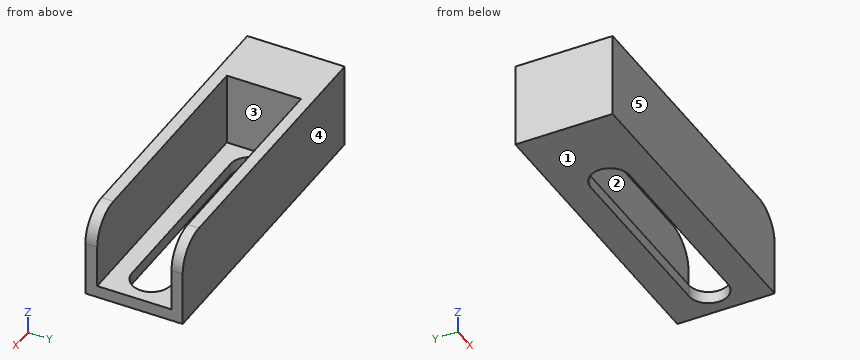
from build123d import *

# Parameters (mm, degrees)
SKETCH_W        = 50
SKETCH_H        = 16
PAD_DEPTH       = 14
SKETCH001_W     = 40
SKETCH001_H     = 12.2
POCKET_DEPTH    = 12
POCKET001_DEPTH = 5
FILLET_R        = 5


with BuildPart() as part:
    # Sketch → Pad (new body)
    with BuildSketch(Plane.XY):
        with Locations((25, 8)):
            Rectangle(SKETCH_W, SKETCH_H)
    extrude(amount=PAD_DEPTH)

    # Sketch001 (on Face6 of Pad) → Pocket (cut)
    with BuildSketch(Plane.XY.offset(14)):
        with Locations((30, 8.058537)):
            Rectangle(SKETCH001_W, SKETCH001_H)
    extrude(amount=-POCKET_DEPTH, mode=Mode.SUBTRACT)

    # Sketch002 (on Face8 of Pocket) → Pocket001 (cut)
    with BuildSketch(Plane.XY.offset(2)):
        with BuildLine():
            ThreePointArc((14.443499, 11.3), (11.243499, 8.1), (14.443499, 4.9))
            Line((14.443499, 4.9), (44.78962, 4.9))
            ThreePointArc((44.78962, 4.9), (47.98962, 8.1), (44.78962, 11.3))
            Line((14.443499, 11.3), (44.78962, 11.3))
        make_face()
    extrude(amount=-POCKET001_DEPTH, mode=Mode.SUBTRACT)

    # Fillet
    fillet_edges = [part.edges().sort_by_distance(p)[0] for p in [
        (50, 0.979269, 14),
        (50, 15.079269, 14),
    ]]
    fillet(fillet_edges, radius=FILLET_R)


solid = part.part
Part model, mm, in its own coordinate system. Face numbers are marked on the shaded views. A direction names the side the tool comes from. Give positions to 0.01 mm unless a question says otherwise; leave off trailing zeros. Order: outer loops, then holes, each group sorted by start corner. A loop starts at its lowest first (then second) coordinate and runs counter-clockwise, first axis right, second up. Notation, with made-up numbers: (-6, -16.75) - (52, -16.75) arc R20 ccw to (52, 16.25) - close; hole circle Ø3 at (19, 81). An arc over 180 degrees is marked (long way). Use a Markdown table: item, result.
1) Two-plate mould, pull along Y, no slides. Class the marked faces 3, 4 and 5: +Y half, -Y half, draft (parallel to the pull), parting line (faces both ways), or undercut.
Checked values:
| item | result |
|---|---|
| face 3 | undercut |
| face 4 | +Y half |
| face 5 | -Y half |
2) Probe L1, parallel to Y at x = 14, z = 9; L2, parallel to X at y = 5, z = 8; L3, parallel to Z at x = 30, y = 2. List the from-to ranges inside material, lowest first. Write a range as from..to.
Checked values:
| item | result |
|---|---|
| L1 | 0..1.96, 14.16..16 |
| L2 | 0..10 |
| L3 | 0..2 |
3) 3-axis set-ups, long thin cutter, end or side, ignore diameter. For the marked faces 1 and 2: which of +Z, -Z, +X, -X, +Y, -Y reach the whole face in a straight line?
Checked values:
| item | result |
|---|---|
| face 1 | -Z, +X, -X, +Y, -Y |
| face 2 | +Z, +X |
4) Saw through at A-A on z = 1. List the corners of the cut face in (x, y), plus the area to 3 significant figures.
Checked values:
| item | result |
|---|---|
| outline | (0, 0) - (50, 0) - (50, 16) - (0, 16) - close; hole (14.44, 4.9) - (44.79, 4.9) arc R3.2 ccw to (44.79, 11.3) - (14.44, 11.3) arc R3.2 ccw to start |
| area | 574 mm² |
5) Saw through at B-B on y = 8.1. List the corners of the cut face in (x, z), plus the area to 3 significant figures.
Checked values:
| item | result |
|---|---|
| outline | (0, 0) - (11.24, 0) - (11.24, 2) - (10, 2) - (10, 14) - (0, 14) - close; (47.99, 0) - (50, 0) - (50, 2) - (47.99, 2) - close |
| area | 147 mm² |
6) Saw through at C-C on x = 19.5. List the corners of the cut face in (y, z), plus the area to 3 significant figures.
Checked values:
| item | result |
|---|---|
| outline | (0, 0) - (4.9, 0) - (4.9, 2) - (1.96, 2) - (1.96, 14) - (0, 14) - close; (11.3, 0) - (16, 0) - (16, 14) - (14.16, 14) - (14.16, 2) - (11.3, 2) - close |
| area | 64.8 mm² |
7) Saw through at D-D on y = 12.25. List the corners of the cut face in (x, z).
Checked values:
| item | result |
|---|---|
| outline | (0, 0) - (50, 0) - (50, 2) - (10, 2) - (10, 14) - (0, 14) - close |
8) Flat gauge pins, fed straight in: P1, Ø3.5, axis at y = 9, z = 6.5, coming from the +X side; P2, Ø3.5, axis at x = 22.5, y = 6.5, coming from the +Z side. Where does each tip first touch, or does it go through?
Checked values:
| item | result |
|---|---|
| P1 | x = 10 |
| P2 | z = 2 |
